```python
from build123d import *

# Parameters (mm, degrees)
F0_R     = 7
F1_DEPTH = 45
F3_DEPTH = 25
F4_R     = 3.65
F5_DEPTH = 10
F7_DEPTH = 4


with BuildPart() as f1:
    # F0 (on Top) → F1 (new body)
    with BuildSketch(Plane.XY):
        Circle(F0_R)
    extrude(amount=F1_DEPTH)

    # F2 (on face) → F3 (cut)
    with BuildSketch(Plane.XY.offset(45)):
        with BuildLine():
            ThreePointArc((4.769696, 1.5), (0, 5), (-4.769696, 1.5))
            Line((-4.769696, 1.5), (-3, 1.5))
            Line((-3, 1.5), (-3, -1.5))
            Line((-3, -1.5), (-4.769696, -1.5))
            ThreePointArc((-4.769696, -1.5), (0, -5), (4.769696, -1.5))
            Line((4.769696, -1.5), (3, -1.5))
            Line((3, -1.5), (3, 1.5))
            Line((3, 1.5), (4.769696, 1.5))
        make_face()
    extrude(amount=-F3_DEPTH, mode=Mode.SUBTRACT)

    # F4 (on face) → F5 (cut)
    with BuildSketch(Plane(origin=(0, 0, 0), x_dir=(1, 0, 0), z_dir=(0, 0, -1))):
        Circle(F4_R)
    extrude(amount=-F5_DEPTH, mode=Mode.SUBTRACT)

    # F6 (on face) → F7 (cut)
    with BuildSketch(Plane(origin=(0, 0, 10), x_dir=(1, 0, 0), z_dir=(0, 0, -1))):
        with BuildLine():
            Line((-1.5, 2), (-1.5, -2))
            ThreePointArc((-1.5, -2), (2.5, 0), (-1.5, 2))
        make_face()
    extrude(amount=-F7_DEPTH, mode=Mode.SUBTRACT)


solid = f1.part
```
Source: CAD feature listing. Evaluate the final solid. Frame: model axes, mm. A direction names the side the tool comes from. Give positions to 0.01 mm unless a question says otherwise; leave off trailing zeros. Loops run counter-clockwise (first coordinate to the right, second up) from the corner with the lowest first, then second, coordinate; pieces in that order, holes last. Notation, with made-up numbers: (51, -8) -> (90, -8) arc R17 ccw to (90, 16) -> close; hole circle Ø8 at (26.25, 46.5). An arc over 180 degrees is marked (long way). Put each result on its own line as item: value. Start each with the question number.
1) Draft query along Y for faces 4 (the face through (6.466, -2.681, 22.185)), 5 (the face through (0, -5, 33)), 6 (the face through (3, -3, 0)), 7 (the face through (3.48, -1.1, 4.93)). Return one class per face: released by +Y, released by -Y, zero draft, split by the parting line, or undercut.
2) Reachability of faces 1 (the face through (-3.2, 0.1, 45)), 2 (the face through (-1.5, 0, 12)), 3 (the face through (4, -1.5, 33)) from +Z, -Z, +X, -X, +Y, -Y: full face, straight path, thin tool, end or side. Return the list, or none.
3) Cut plane B-B (z = 20.5). Return loops of the section in (x, y).
4) Cut plane A-A (x = 0). Return loops of the section in (y, z), then the cut area to 3 significant figures.
5) Cut plane C-C (y = 0). Return loops of the section in (x, z).
6) Material intervals for probe 1 along Y at (x, z) = (0, 2.5); probe 2 along Y at (x, z) = (0, 11); probe 3 along Y at (x, z) = (3.25, 25), sorted ascending.
7) Cut plane D-D (z = 13). Return loops of the section in (x, y), then the cut area to 3 significant figures.
8) Contact query for flat-ended pins moving along their axis: P1, Ø1.4, axis at x = 4, z = 35, coming from the +Y side; P2, Ø1.5, axis at y = 3, z = 34.5, coming from the -X side; P3, Ø4, axis at x = -3, z = 24.5, coming from the +Y side. Output: stop coordinate, or through.
Results are:
1. face 4: split by the parting line
1. face 5: undercut
1. face 6: zero draft
1. face 7: undercut
2. face 1: +Z, +X, -X, +Y, -Y
2. face 2: -Z
2. face 3: +Z
3. outline: circle Ø14 at (0, 0); hole (-4.77, -1.5) arc R5 ccw to (4.77, -1.5) -> (3, -1.5) -> (3, 1.5) -> (4.77, 1.5) arc R5 ccw to (-4.77, 1.5) -> (-3, 1.5) -> (-3, -1.5) -> close
4. outline: (-7, 0) -> (-3.65, 0) -> (-3.65, 10) -> (-2.5, 10) -> (-2.5, 14) -> (2.5, 14) -> (2.5, 10) -> (3.65, 10) -> (3.65, 0) -> (7, 0) -> (7, 45) -> (5, 45) -> (5, 20) -> (-5, 20) -> (-5, 45) -> (-7, 45) -> close
4. area: 287 mm2
5. outline: (-7, 0) -> (-3.65, 0) -> (-3.65, 10) -> (-1.5, 10) -> (-1.5, 14) -> (2.5, 14) -> (2.5, 10) -> (3.65, 10) -> (3.65, 0) -> (7, 0) -> (7, 45) -> (3, 45) -> (3, 20) -> (-3, 20) -> (-3, 45) -> (-7, 45) -> close
6. probe 1: y = -7 to -3.65, 3.65 to 7
6. probe 2: y = -7 to -2.5, 2.5 to 7
6. probe 3: y = -6.2 to -3.8, -1.5 to 1.5, 3.8 to 6.2
7. outline: circle Ø14 at (0, 0); hole (-1.5, -2) arc R2.5 ccw (long way) to (-1.5, 2) -> close
7. area: 137 mm2
8. P1: stops at y = 6.17
8. P2: stops at x = -6.63
8. P3: stops at y = 6.93
